Build history of the part. All positions in model axes, mm. Face numbers are marked on the shaded views. Round coordinates to 2 decimals unless told otherwise and drop trailing zeros. Order: outer loops, then holes, each group sorted by start corner. A loop starts at its lowest first (then second) coordinate and runs counter-clockwise, first axis right, second up. Notation, with made-up numbers: (0, 78) -> (28, 78) arc R26 cw to (28, 107) -> close; hole circle Ø7 at (-5.75, -20.75). An arc over 180 degrees is marked (long way). Use a Markdown table: item, result. Add a question column.
Item 1: Slice it at B-B, the plane z = -101. Give the cut face in (x, y).
Item 2: Slice it at D-D, the plane y = 195. Give the cut face in (x, z).
Item 3: Pin check, flat tips, straight feed: pin 1 (2.5 mm diameter, centred on y = 206.5, z = -212, fed in from +X); pin 2 (9.5 mm diameter, centred on x = -60.5, z = -150.8, fed in from -Y); pin 3 (5 mm diameter, centred on y = 205.5, z = -169, fed in from -X). Stop position of each tip, or through.
Item 4: Two-plate mould, pull along X, no slides. Class the marked faces 1 and 2: released by +X, released by -X, zero draft, split by the parting line, or undercut.
Item 5: Slice it at A-A, the plane z = -230.8. Give the cut face in (x, y), plus the area to 3 significant figures.
Item 6: Probe L1, parallel to X at y = 191.75, z = -262; L2, parallel to X at y = 203, z = -227; L3, parallel to Y at x = -75.5, z = -19. List the from-to ranges inside material, lowest first.
Item 7: Slice it at C-C, the plane z = -150.8. Give the cut face in (x, y), plus the area to 3 significant figures.
from build123d import *

# Parameters (mm, degrees)
SKETCH1_W                   = 70
SKETCH1_H                   = 290
BASE_FLANGE1_DEPTH          = 3
SM_EDGE_FLANGE_1_DEPTH      = 290
SM_EDGE_FLANGE_1_BEND_DEPTH = 290
INDENT1_START               = -127
INDENT1_DEPTH               = 84
INDENT1_START_2             = -123.729611107
INDENT1_2_DEPTH             = 77.459222009
INDENT1_3_DEPTH             = 0.729611107
INDENT1_START_3             = -47
INDENT1_4_DEPTH             = 0.729610902
INDENT1_START_4             = -50.0000001
INDENT1_5_DEPTH             = 6.0000001
INDENT1_START_5             = -126
INDENT1_6_DEPTH             = 6
INDENT1_START_6             = -290
INDENT1_7_DEPTH             = 6.65
INDENT2_START               = -127
INDENT2_DEPTH               = 84
INDENT2_START_2             = -11.0000001
INDENT2_2_DEPTH             = 11.0000001
INDENT2_START_3             = -126
INDENT2_3_DEPTH             = 82
CUT_EXTRUDE1_DEPTH          = 317.754179273
CUT_EXTRUDE1_DEPTH_BACK     = 317.754179273
SKETCH12_R                  = 4.2
CUT_EXTRUDE2_DEPTH          = 10


with BuildPart() as part:
    # Base-Flange1: sheet metal written as solids
    # Sketch1 → Base-Flange1 (new body)
    with BuildSketch(Plane(origin=(0, 207.95, 0), x_dir=(1, 0, 0), z_dir=(0, 1, 0))):
        with Locations((-85, 145)):
            Rectangle(SKETCH1_W, SKETCH1_H)
    extrude(amount=-BASE_FLANGE1_DEPTH)

    # 邊線-凸緣1: sheet metal written as solids
    # 邊線-凸緣1 section (on a plane across the edge) → 邊線-凸緣1 (add)
    with BuildSketch(Plane(origin=(-47, 204.95, -290), x_dir=(-1, 0, 0), z_dir=(0, 0, 1))):
        with BuildLine():
            Line((-3, 3), (-3, 15.9))
            Line((-3, 15.9), (0, 15.9))
            Line((0, 15.9), (0, 3))
            ThreePointArc((0, 3), (0.878679656, 0.878679656), (3, 0))
            Line((3, 0), (3, -3))
            ThreePointArc((3, -3), (-1.242640687, -1.242640687), (-3, 3))
        make_face()
    extrude(amount=SM_EDGE_FLANGE_1_DEPTH)

    # 邊線-凸緣1 section 2 (on a plane across the edge) → 邊線-凸緣1 bend (add)
    with BuildSketch(Plane(origin=(-123, 204.95, 0), x_dir=(1, 0, 0), z_dir=(0, 0, -1))):
        with BuildLine():
            Line((-3, 3), (-3, 15.9))
            Line((-3, 15.9), (0, 15.9))
            Line((0, 15.9), (0, 3))
            ThreePointArc((0, 3), (0.878679656, 0.878679656), (3, 0))
            Line((3, 0), (3, -3))
            ThreePointArc((3, -3), (-1.242640687, -1.242640687), (-3, 3))
        make_face()
    extrude(amount=SM_EDGE_FLANGE_1_BEND_DEPTH)

    # Indent1: read off the stored shape, not the designer's step
    # Indent1 outline → Indent1 (cut)
    with BuildSketch(Plane.YZ.offset(INDENT1_START)):
        with BuildLine():
            Line((192.05, -290), (207.95, -290))
            ThreePointArc((207.95, -290), (200, -282.05), (192.05, -290))
        make_face()
    extrude(amount=INDENT1_DEPTH, mode=Mode.SUBTRACT)

    # Indent2: read off the stored shape, not the designer's step
    # Indent2 outline → Indent2 (cut)
    with BuildSketch(Plane.YZ.offset(INDENT2_START)):
        with BuildLine():
            ThreePointArc((189.05, -6.433311744), (197.7062633, -12.491147744), (207.950014124, -9.903902031))
            Line((207.950014124, -9.903902031), (209, -9.061062257))
            Line((209, -9.061062257), (209, 1))
            Line((209, 1), (188, 1))
            Line((188, 1), (188, 0))
            Line((188, 0), (188, -4.64612958))
            Line((188, -4.64612958), (189.05, -6.433311744))
        make_face()
    extrude(amount=INDENT2_DEPTH, mode=Mode.SUBTRACT)

    # Sketch12 → Cut-Extrude1 (cut, two sides: drawn at the far end of the back side and taken through both)
    with BuildSketch(Plane(origin=(0, 207.95, 0), x_dir=(1, 0, 0), z_dir=(0, 1, 0)).offset(-CUT_EXTRUDE1_DEPTH_BACK)):
        with Locations((-109.5, 270.8)):
            Circle(SKETCH12_R)
        with Locations((-60.5, 270.8)):
            Circle(SKETCH12_R)
        with Locations((-60.5, 250.8)):
            Circle(SKETCH12_R)
        with Locations((-109.5, 250.8)):
            Circle(SKETCH12_R)
        with Locations((-60.5, 230.8)):
            Circle(SKETCH12_R)
        with Locations((-109.5, 230.8)):
            Circle(SKETCH12_R)
        with Locations((-60.5, 210.8)):
            Circle(SKETCH12_R)
        with Locations((-109.5, 210.8)):
            Circle(SKETCH12_R)
        with Locations((-60.5, 190.8)):
            Circle(SKETCH12_R)
        with Locations((-109.5, 190.8)):
            Circle(SKETCH12_R)
        with Locations((-60.5, 170.8)):
            Circle(SKETCH12_R)
        with Locations((-109.5, 170.8)):
            Circle(SKETCH12_R)
        with Locations((-60.5, 150.8)):
            Circle(SKETCH12_R)
        with Locations((-109.5, 150.8)):
            Circle(SKETCH12_R)
        with Locations((-60.5, 130.8)):
            Circle(SKETCH12_R)
        with Locations((-109.5, 130.8)):
            Circle(SKETCH12_R)
        with Locations((-60.5, 110.8)):
            Circle(SKETCH12_R)
        with Locations((-109.5, 110.8)):
            Circle(SKETCH12_R)
    extrude(amount=CUT_EXTRUDE1_DEPTH + CUT_EXTRUDE1_DEPTH_BACK, mode=Mode.SUBTRACT)

    # Sketch13 → Cut-Extrude2 (cut)
    with BuildSketch(Plane(origin=(0, 207.95, 0), x_dir=(1, 0, 0), z_dir=(0, 1, 0))):
        with BuildLine():
            Line((-70, 107.7), (-70, 42.7))
            ThreePointArc((-70, 42.7), (-85, 27.7), (-100, 42.7))
            Line((-100, 42.7), (-100, 107.7))
            ThreePointArc((-100, 107.7), (-85, 122.7), (-70, 107.7))
        make_face()
        with BuildLine():
            Line((-70, 245), (-70, 180))
            ThreePointArc((-70, 180), (-85, 165), (-100, 180))
            Line((-100, 180), (-100, 245))
            ThreePointArc((-100, 245), (-85, 260), (-70, 245))
        make_face()
    extrude(amount=-CUT_EXTRUDE2_DEPTH, mode=Mode.SUBTRACT)


with BuildPart() as body_2:
    # Indent1 2 outline → Indent1 2 (new body)
    with BuildSketch(Plane.YZ.offset(INDENT1_START_2)):
        with BuildLine():
            Line((204.95, -285.559279338), (204.95, -290))
            Line((204.95, -290), (206.65, -290))
            ThreePointArc((206.65, -290), (206.210475022, -287.622501314), (204.95, -285.559279338))
        make_face()
    extrude(amount=INDENT1_2_DEPTH)

    # Indent1 3 outline → Indent1 3 (add)
    with BuildSketch(Plane.YZ.offset(INDENT1_START_2)):
        with BuildLine():
            Line((193.35, -290), (204.95, -290))
            Line((204.95, -290), (204.95, -285.559279338))
            ThreePointArc((204.95, -285.559279338), (197.622501314, -283.789524978), (193.35, -290))
        make_face()
    extrude(amount=INDENT1_3_DEPTH)

    # Indent1 4 outline → Indent1 4 (add)
    with BuildSketch(Plane.YZ.offset(INDENT1_START_3)):
        with BuildLine():
            Line((193.35, -290), (204.95, -290))
            Line((204.95, -290), (204.95, -285.559279338))
            ThreePointArc((204.95, -285.559279338), (197.622501314, -283.789524978), (193.35, -290))
        make_face()
    extrude(amount=INDENT1_4_DEPTH)

    # Indent1 5 outline → Indent1 5 (add)
    with BuildSketch(Plane.YZ.offset(INDENT1_START_4)):
        with BuildLine():
            Line((193.35, -290), (206.65, -290))
            ThreePointArc((206.65, -290), (200, -283.35), (193.35, -290))
        make_face()
    extrude(amount=INDENT1_5_DEPTH)

    # Indent1 6 outline → Indent1 6 (add)
    with BuildSketch(Plane.YZ.offset(INDENT1_START_5)):
        with BuildLine():
            Line((193.35, -290), (206.65, -290))
            ThreePointArc((206.65, -290), (200, -283.35), (193.35, -290))
        make_face()
    extrude(amount=INDENT1_6_DEPTH)

    # Indent1 7 outline → Indent1 7 (cut)
    with BuildSketch(Plane.XY.offset(INDENT1_START_6)):
        with BuildLine():
            Line((-47, 192), (-47, 201.95))
            ThreePointArc((-47, 201.95), (-47.878679656, 204.071320344), (-50, 204.95))
            Line((-50, 204.95), (-50.0000001, 192))
            Line((-50.0000001, 192), (-47, 192))
        make_face()
        with BuildLine():
            Line((-123, 192), (-120, 192))
            Line((-120, 192), (-120, 204.95))
            ThreePointArc((-120, 204.95), (-122.121320344, 204.071320344), (-123, 201.95))
            Line((-123, 201.95), (-123, 192))
        make_face()
        with BuildLine():
            ThreePointArc((-46.270396534, 206.650006169), (-44.597333029, 204.559825589), (-44, 201.95))
            Line((-44, 201.95), (-44, 208))
            Line((-44, 208), (-47.971644239, 208))
            Line((-47.971644239, 208), (-46.270396534, 206.650006169))
        make_face()
        with BuildLine():
            Line((-126, 208), (-126, 201.95))
            ThreePointArc((-126, 201.95), (-125.402668364, 204.559822705), (-123.729608483, 206.650002187))
            Line((-123.729608483, 206.650002187), (-122.028359489, 208))
            Line((-122.028359489, 208), (-126, 208))
        make_face()
    extrude(amount=INDENT1_7_DEPTH, mode=Mode.SUBTRACT)


with BuildPart() as body_3:
    # Indent2 2 outline → Indent2 2 (new body)
    with BuildSketch(Plane.XY.offset(INDENT2_START_2)):
        with BuildLine():
            Line((-44, 189.05), (-44, 201.95))
            ThreePointArc((-44, 201.95), (-45.757359313, 206.192640687), (-50, 207.95))
            Line((-50, 207.95), (-120, 207.95))
            ThreePointArc((-120, 207.95), (-124.242640687, 206.192640687), (-126, 201.95))
            Line((-126, 201.95), (-126, 189.05))
            Line((-126, 189.05), (-123, 189.05))
            Line((-123, 189.05), (-123, 201.95))
            ThreePointArc((-123, 201.95), (-122.121320344, 204.071320344), (-120, 204.95))
            Line((-120, 204.95), (-50, 204.95))
            ThreePointArc((-50, 204.95), (-47.878679656, 204.071320344), (-47, 201.95))
            Line((-47, 201.95), (-47, 189.05))
            Line((-47, 189.05), (-44, 189.05))
        make_face()
    extrude(amount=INDENT2_2_DEPTH)

    # Indent2 3 outline → Indent2 3 (cut)
    with BuildSketch(Plane.YZ.offset(INDENT2_START_3)):
        with BuildLine():
            Line((207.95, -11.0000001), (207.950016725, -7.602449216))
            ThreePointArc((207.950016725, -7.602449216), (204.322791843, -10.115012145), (200.000000001, -11))
            Line((200.000000001, -11), (207.95, -11.0000001))
        make_face()
        with BuildLine():
            Line((189.05, -11.0000001), (200.000000001, -11))
            ThreePointArc((200.000000001, -11), (192.601479194, -8.140140655), (189.05, -1.047616342))
            Line((189.05, -1.047616342), (189.05, -11.0000001))
        make_face()
    extrude(amount=INDENT2_3_DEPTH, mode=Mode.SUBTRACT)


solid = part.part
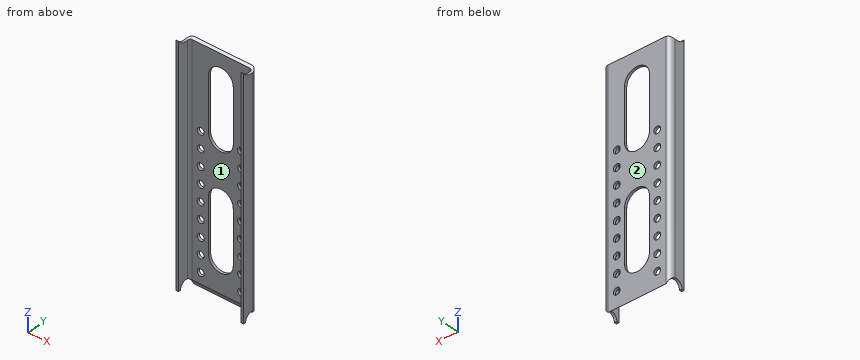
Check sheet entries:
| question | item | result |
|---|---|---|
| 1 | outline | (-126, 189.05) -> (-123, 189.05) -> (-123, 201.95) arc R3 cw to (-120, 204.95) -> (-100, 204.95) -> (-100, 207.95) -> (-120, 207.95) arc R6 ccw to (-126, 201.95) -> close; (-70, 204.95) -> (-50, 204.95) arc R3 cw to (-47, 201.95) -> (-47, 189.05) -> (-44, 189.05) -> (-44, 201.95) arc R6 ccw to (-50, 207.95) -> (-70, 207.95) -> close |
| 2 | outline | (-126, -283.82) -> (-123, -283.82) -> (-123, -11.67) -> (-126, -11.67) -> close; (-47, -283.82) -> (-44, -283.82) -> (-44, -11.67) -> (-47, -11.67) -> close |
| 3 | pin 1 | x = -44.99 |
| 3 | pin 2 | y = 204.95 |
| 3 | pin 3 | x = -125.91 |
| 4 | face 1 | undercut |
| 4 | face 2 | zero draft |
| 5 | outline | (-126, 189.05) -> (-123, 189.05) -> (-123, 201.95) arc R3 cw to (-120, 204.95) -> (-113.7, 204.95) -> (-113.7, 207.95) -> (-120, 207.95) arc R6 ccw to (-126, 201.95) -> close; (-105.3, 204.95) -> (-100, 204.95) -> (-100, 207.95) -> (-105.3, 207.95) -> close; (-70, 204.95) -> (-64.7, 204.95) -> (-64.7, 207.95) -> (-70, 207.95) -> close; (-56.3, 204.95) -> (-50, 204.95) arc R3 cw to (-47, 201.95) -> (-47, 189.05) -> (-44, 189.05) -> (-44, 201.95) arc R6 ccw to (-50, 207.95) -> (-56.3, 207.95) -> close |
| 5 | area | 189 mm2 |
| 6 | L1 | -126 to -123, -47 to -44 |
| 6 | L2 | -125.91 to -122.81, -47.19 to -44.09 |
| 6 | L3 | 204.95 to 207.95 |
| 7 | outline | (-126, 189.05) -> (-123, 189.05) -> (-123, 201.95) arc R3 cw to (-120, 204.95) -> (-113.7, 204.95) -> (-113.7, 207.95) -> (-120, 207.95) arc R6 ccw to (-126, 201.95) -> close; (-105.3, 204.95) -> (-64.7, 204.95) -> (-64.7, 207.95) -> (-105.3, 207.95) -> close; (-56.3, 204.95) -> (-50, 204.95) arc R3 cw to (-47, 201.95) -> (-47, 189.05) -> (-44, 189.05) -> (-44, 201.95) arc R6 ccw to (-50, 207.95) -> (-56.3, 207.95) -> close |
| 7 | area | 279 mm2 |
